Autodesk Inventor part; units mm, degrees
ref_plane "YZ Plane" through (0, 0, 0) normal (1, 0, 0) x (0, 1, 0)
ref_plane "XZ Plane" through (0, 0, 0) normal (0, 1, 0) x (-1, 0, 0)
ref_plane "XY Plane" through (0, 0, 0) normal (0, 0, 1) x (1, 0, 0)
sketch "Эскиз1" plane through (0, 0, 0) normal (1, 0, 0) x (0, 1, 0)
  line L0 (-8.3221, -24.9171) -> (-8.3221, 15.0829)
  line L1 (-8.3221, 15.0829) -> (31.6779, 15.0829)
  arc A0 (-8.3221, -24.9171) -> (31.6779, 15.0829) centre (-8.3221, 15.0829) ccw
  point P0 (0, 0)
  dimension "d1" = 40
extrude "Выдавливание1" add sketch "Эскиз1" along normal mid plane 455
sketch "Эскиз3" plane through (-227.5, -8.3221, 15.0829) normal (0, 0, 1) x (1, 0, 0)
  line L0 (0, 0) -> (455, 0)
  line L1 (455, 40) -> (455, 0)
  line L2 (455, 40) -> (0, 40)
  line L3 (0, 0) -> (0, 40)
  point P0 (227.5, 8.3221)
extrude "Выдавливание2" add sketch "Эскиз3" along normal blind 30
sketch "Эскиз4" plane through (-227.5, 31.6779, 15.0829) normal (0, 1, 0) x (1, 0, 0)
  line L0 (455, 0) -> (0, 0)
  line L1 (0, 0) -> (0, -30)
  line L2 (455, -30) -> (0, -30)
  line L3 (455, 0) -> (455, -30)
  point P0 (227.5, 15.0829)
extrude "Выдавливание3" cut sketch "Эскиз4" against normal blind 4
sketch "Эскиз6" plane through (-227.5, 27.6779, 15.0829) normal (0, 1, 0) x (1, 0, 0)
  line L0 (0, 40) -> (0, -30)
  line L1 (0, -14.536) -> (200.0528, -14.536) construction
  line L2 (455, 0) -> (0, 0)
  circle A0 centre (10.061, -14.536) radius 8.0645
  circle A1 centre (37.061, -14.536) radius 8.0645
  circle A2 centre (64.061, -14.536) radius 8.0645
  circle A3 centre (91.061, -14.536) radius 8.0645
  circle A4 centre (118.061, -14.536) radius 8.0645
  circle A5 centre (145.061, -14.536) radius 8.0645
  circle A6 centre (172.061, -14.536) radius 8.0645
  point P0 (227.5, 15.0829)
  dimension "d21" = 14.536
  dimension "d22" = 16.129
  dimension "d23" = 10.061
  dimension "d26" = 27
extrude "Выдавливание5" [suppressed]
sketch "Эскиз8" plane through (-227.5, -8.3221, -24.9171) normal (0, -1, 0) x (1, 0, 0)
  line L0 (455, 50) -> (465, 55)
  line L1 (465, 55) -> (465, 35)
  line L2 (465, 35) -> (455, 40)
  line L3 (455, 0) -> (455, 70)
  point P0 (227.5, 24.9171)
  point P1 (465, 45)
  dimension "d33" = 20
  dimension "d34" = 10
  dimension "d35" = 20
  dimension "d36" = 15
  dimension "d37" = 10
extrude "Выдавливание6" [suppressed]
sketch "Эскиз9" plane through (-227.5, -8.3221, -24.9171) normal (0, -1, 0) x (1, 0, 0)
  line L0 (210, 40) -> (220, 45)
  line L1 (220, 45) -> (220, 25)
  line L2 (220, 25) -> (210, 30)
  line L3 (455, 0) -> (455, 70)
  line L4 (-10, 25) -> (-10, 45)
  line L5 (-10, 45) -> (0, 40)
  line L6 (0, 30) -> (-10, 25)
  line L7 (0, 0) -> (0, 70)
  point P0 (227.5, 24.9171)
extrude "Выдавливание7" [suppressed]
sketch "Эскиз10" plane through (-227.5, -8.3221, -24.9171) normal (0, -1, 0) x (1, 0, 0)
  line L0 (-10, 45) -> (0, 40)
  line L1 (-10, 25) -> (-10, 45)
  line L2 (0, 30) -> (-10, 25)
  line L3 (0, 0) -> (0, 70)
  point P0 (227.5, 24.9171)
extrude "Выдавливание8" add sketch "Эскиз10" against normal blind 20
sketch "Эскиз11" plane through (-227.5, -8.3221, -24.9171) normal (0, -1, 0) x (1, 0, 0)
  line L0 (0, 70) -> (455, 70)
  line L1 (0, 0) -> (455, 0)
  line L2 (0, 40) -> (455, 40)
  point P0 (227.5, 24.9171)
feature "Разделение1" [suppressed]
sketch "Эскиз14" plane through (-227.5, 27.6779, 15.0829) normal (0, 1, 0) x (1, 0, 0)
  line L0 (0, 0) -> (455, 0)
  line L1 (0, -30) -> (455, -30)
  line L2 (134.048, 0) -> (100.336, 0)
  line L3 (100.336, 0) -> (100.336, -30) construction
  line L4 (100.336, -30) -> (134.048, -30)
  line L5 (134.048, -30) -> (134.048, 0)
  line L6 (105, 0) -> (105, -320)
  line L7 (319.048, 0) -> (285.336, 0)
  line L8 (285.336, -30) -> (319.048, -30)
  line L9 (319.048, -30) -> (319.048, 0)
  line L10 (290, 0) -> (290, -320)
  point P0 (227.5, 15.0829)
  point P1 (105, -30)
  point P2 (134.048, -30)
  point P3 (290, -30)
  point P4 (319.048, -30)
  dimension "d71" = 33.712
  dimension "d72" = 4.664
  dimension "d75" = 185
extrude "Выдавливание10" [suppressed]
ref_plane "РабПлоскость1" through (-227.5, 31.6779, 30.0829) normal (0, 0, 1) x (1, 0, 0)
sketch "Эскиз16" plane through (-227.5, -8.3221, -24.9171) normal (0, -1, 0) x (1, 0, 0)
  circle A0 centre (115, 55) radius 2.529
  line L0 (-91, 55) -> (546, 55) construction
  line L1 (115, 360) -> (115, 40) construction
  line L2 (300, 360) -> (300, 40) construction
  circle A1 centre (300, 55) radius 2.529
  point P0 (227.5, 24.9171)
  dimension "d82" = 5.058
extrude "Выдавливание11" [suppressed]
sketch "Эскиз12" plane through (-227.5, 27.6779, 15.0829) normal (0, 1, 0) x (1, 0, 0)
  line L0 (0, 0) -> (455, 0)
  line L1 (248.041, 0) -> (248.041, -5)
  line L2 (248.041, -5) -> (264.217, -4.95)
  line L3 (264.217, -4.95) -> (264.217, -17.926)
  line L4 (264.217, -17.926) -> (248.041, -20.945)
  line L5 (248.041, -20.945) -> (248.041, -30)
  line L6 (0, -30) -> (455, -30)
  line L7 (227.5, 54) -> (227.5, -44)
  point P0 (227.5, 15.0829)
  dimension "d54" = 20.541
  dimension "d55" = 16.176
  dimension "d56" = 12.074
  dimension "d57" = 4.95
  dimension "d58" = 9.055
  dimension "d59" = 5
feature "Разделение2" [suppressed]
sketch "Эскиз13" plane through (-227.5, 27.6779, 15.0829) normal (0, 1, 0) x (1, 0, 0)
  line L0 (0, -30) -> (455, -30)
  line L1 (0, 0) -> (455, 0)
  line L2 (346, -30) -> (324, -30)
  line L3 (324, -30) -> (324, 0)
  line L4 (324, 0) -> (346, 0)
  line L5 (346, 0) -> (346, -30)
  line L6 (325, -320) -> (325, 0)
  line L7 (161, -30) -> (139, -30)
  line L8 (139, -30) -> (139, 0)
  line L9 (139, 0) -> (161, 0)
  line L10 (161, 0) -> (161, -30)
  point P0 (227.5, 15.0829)
  point P1 (325, -30)
  point P2 (346, 0)
  point P3 (161, 0)
  dimension "d60" = 22
  dimension "d61" = 1
  dimension "d66" = 185
extrude "Выдавливание9" cut sketch "Эскиз13" against normal blind 21 contours L8 L1 L10 L0 | L6 L1 L5 L0
sketch "Эскиз17" plane through (-227.5, -8.3221, -24.9171) normal (0, -1, 0) x (1, 0, 0)
  circle A0 centre (150, 55) radius 2.1
  line L0 (-91, 55) -> (546, 55) construction
  line L1 (150, 40) -> (150, 360) construction
  line L2 (335, 40) -> (335, 360) construction
  circle A1 centre (335, 55) radius 2.1
  point P0 (227.5, 24.9171)
  dimension "d85" = 4.2
extrude "Выдавливание12" cut sketch "Эскиз17" against normal up to next
sketch "Эскиз18" plane through (-227.5, 0, 0) normal (-1, 0, 0) x (0, 0, 1)
  arc A0 (15.0829, 17.6779) -> (-10.9171, -8.3221) centre (15.0829, -8.3221) ccw
  line L0 (-24.9171, -8.3221) -> (45.0829, -8.3221)
  arc A1 (15.0829, 27.6779) -> (-20.9171, -8.3221) centre (15.0829, -8.3221) ccw construction
  line L1 (45.0829, 27.6779) -> (15.0829, 27.6779)
  line L2 (15.0829, 17.6779) -> (15.0829, 27.6779) construction
  line L3 (45.0829, -8.3221) -> (45.0829, 27.6779)
  arc A2 (15.6159, 17.1393) -> (-10.3841, -8.3221) centre (15.0829, -8.3221) ccw
  line L4 (15.6159, 17.1393) -> (15.6159, 28.207)
  arc A3 (15.6159, 28.207) -> (-21.4501, -8.3221) centre (15.0829, -8.3221) ccw
  point P0 (0, 0)
  point P1 (15.0829, 17.6779)
  point P2 (-21.4501, -8.3221)
  point P3 (-10.3841, -8.3221)
  dimension "d94" = 0.533
extrude "Выдавливание13" [suppressed]
sketch "Эскиз19" plane through (-227.5, 27.6779, 15.0829) normal (0, 1, 0) x (1, 0, 0)
  line L0 (237.5, 0) -> (0, 0)
  line L1 (105, -30) -> (0, -30)
  line L2 (0, 0) -> (16.614, 0)
  line L3 (16.614, 0) -> (16.614, -30)
  line L4 (16.614, -30) -> (0, -30)
  line L5 (0, -30) -> (0, 0)
  point P0 (227.5, 15.0829)
  dimension "d90" = 16.614
extrude "Выдавливание14" [suppressed]
properties part number "Край задней части корпуса"
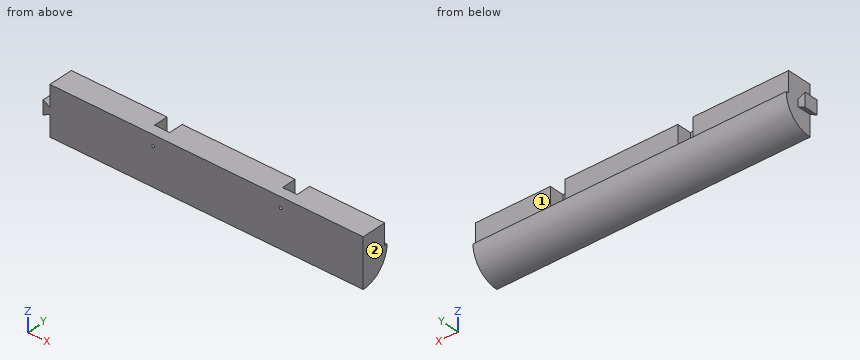
Could you check a few things on this model? Use its own coordinates, in mm. Face numbers are marked on the shaded views. A direction names the side the tool comes from. Round coordinates to 2 decimals unless told otherwise and drop trailing zeros. Write each loop counter-clockwise with the first axis right and the second up, starting at its lowest first coordinate (ties: lowest second). Pieces come first, ordered by that corner, then holes. Notation, with made-up numbers: (-37, 21) -> (15, 21) arc R32 cw to (15, 58) -> close; hole circle Ø1 at (4, 79). An arc over 180 degrees is marked (long way). Use a Markdown table: item, result.
1. If we section it at B-B (y = 20.5): List the corners of the cut face in (x, z) for me, then the cut area to 3 significant figures.
Answer key:
| item | result |
|---|---|
| outline | (-227.5, -12.65) -> (227.5, -12.65) -> (227.5, 45.08) -> (118.5, 45.08) -> (118.5, 15.08) -> (97.5, 15.08) -> (97.5, 45.08) -> (-66.5, 45.08) -> (-66.5, 15.08) -> (-88.5, 15.08) -> (-88.5, 45.08) -> (-227.5, 45.08) -> close |
| area | 25,000 mm^2 |
2. Please list where these lines run through material, in increasing order: probe 1 along X at (y, z) = (15.5, 28); probe 2 along X at (y, z) = (-3.5, 34); probe 3 along X at (y, z) = (-1.5, 15.5).
Answer key:
| item | result |
|---|---|
| probe 1 | x = -227.5 to -88.5, -66.5 to 97.5, 118.5 to 227.5 |
| probe 2 | x = -227.5 to 227.5 |
| probe 3 | x = -237.5 to -228.33, -227.5 to 227.5 |
3. If we section it at A-A (x = -3): List the corners of the cut face in (y, z) for me.
Answer key:
| item | result |
|---|---|
| outline | (-8.32, -24.92) arc R40 ccw to (31.68, 15.08) -> (27.68, 15.08) -> (27.68, 45.08) -> (-8.32, 45.08) -> close |
4. Which directions (+Z, -Z, +X, -X, +Y, -Y) give clear straight access to the entire face, cutting with the end or side of a thin tool? Please do the marked faces 1 and 2.
Answer key:
| item | result |
|---|---|
| face 1 | +Z, +X, -X, +Y |
| face 2 | +Z, -Z, +X, +Y, -Y |
5. For pin 1 Ø15 at (x, z) = (-124, 29) entering from +Y; pin 2 Ø6.5 at (y, z) = (13.5, 30) entering from -X; pin 3 Ø5 at (x, z) = (-231, 7.5) entering from +Y; pin 4 Ø6.5 at (x, z) = (-77.5, 30.08) entering from -Y, each with a flat end and sliding along its axis, tell me the tip position at first contact or that it passes through.
Answer key:
| item | result |
|---|---|
| pin 1 | stops at y = 27.68 |
| pin 2 | stops at x = -227.5 |
| pin 3 | stops at y = 11.68 |
| pin 4 | stops at y = -8.32 |
